Input: part model. Units: mm. Frame: model coordinates. Coordinates: 2 decimals unless noted, no trailing zeros. Loops run counter-clockwise (first coordinate to the right, second up) from the corner with the lowest first, then second, coordinate; pieces in that order, holes last. Notation, with made-up numbers: M -15.5,25 L 16.5,25 A28 ccw 16.5,47 Z; hole C 70,31 d2. An arc over 180 degrees is marked long. Use a Markdown table: item, result. Add a question column.
1. Draft query along Z for faces 1 (the flat face through (-54, 0, 2)), 2 (the cylindrical face through (-75.63, 0.69, 14.27)), 3 (the cylindrical face through (-61.554, 0.69, -13.226)). Return one class per face: +Z half, -Z half, draft (parallel to the pull), parting line (faces both ways), or undercut.
2. Section B-B on x = -63.5. Output: boundary loops of the cut face in (y, z), then the cut area to 3 significant figures.
3. Pin query (flat end, axial travel): pin 1 (1.9 mm diameter, centred on x = -62.65, z = 16.29, fed in from +Y). Return the tip coordinate at first contact, or that it passes through.
4. Line query: L1, parallel to X at y = 1, z = -13; L2, parallel to X at y = 1.2, z = 15; L3, parallel to Z at x = -60, y = 1.35. Output: solid intervals per line, ascending. Write a range as [from, to].
5. Section D-D on z = 21. Output: boundary loops of the cut face in (x, y), then the cut area to 3 significant figures.
6. Section C-C on y = 1.05. Output: boundary loops of the cut face in (x, z), then the cut area to 3 significant figures.
7. Section A-A on z = -14. Output: boundary loops of the cut face in (x, y).
Autodesk Inventor part; units mm, degrees
ref_plane "YZ Plane" through (0, 0, 0) normal (1, 0, 0) x (0, 1, 0)
ref_plane "XZ Plane" through (0, 0, 0) normal (0, 1, 0) x (-1, 0, 0)
ref_plane "XY Plane" through (0, 0, 0) normal (0, 0, 1) x (1, 0, 0)
sketch "Sketch1" plane through (0, 0, 0) normal (0, 1, 0) x (-1, 0, 0)
  line L0 (55.4027, 26.2487) -> (74.9027, 14.9904)
  line L1 (75.9027, 13.2583) -> (75.9027, -9.2583)
  line L2 (74.9027, -10.9904) -> (55.4027, -22.2487)
  line L3 (53.4027, -22.2487) -> (33.9027, -10.9904)
  line L4 (32.9027, -9.2583) -> (32.9027, 13.2583)
  line L5 (33.9027, 14.9904) -> (53.4027, 26.2487)
  arc A0 (33.9027, 14.9904) -> (32.9027, 13.2583) centre (34.9027, 13.2583) ccw
  arc A1 (32.9027, -9.2583) -> (33.9027, -10.9904) centre (34.9027, -9.2583) ccw
  arc A2 (53.4027, -22.2487) -> (55.4027, -22.2487) centre (54.4027, -20.5167) ccw
  arc A3 (74.9027, -10.9904) -> (75.9027, -9.2583) centre (73.9027, -9.2583) ccw
  arc A4 (75.9027, 13.2583) -> (74.9027, 14.9904) centre (73.9027, 13.2583) ccw
  arc A5 (55.4027, 26.2487) -> (53.4027, 26.2487) centre (54.4027, 24.5167) ccw
  circle A6 centre (63.1527, -13.1554) radius 1.6
  circle A7 centre (62.6527, 16.2894) radius 1.6
  point P0 (0, 0)
  point P1 (54.4027, 26.8261)
  point P2 (75.9027, 14.413)
  point P3 (75.9027, -10.413)
  point P4 (54.4027, -22.8261)
  point P5 (32.9027, -10.413)
  point P6 (32.9027, 14.413)
  dimension "d0" = 3.2
  dimension "d1" = 3.2
extrude "Extrusion1" add sketch "Sketch1" along normal blind 1.4
properties part number "Kicker PCB"
Answers below:
| question | item | result |
|---|---|---|
| 1 | face 1 | draft |
| 1 | face 2 | +Z half |
| 1 | face 3 | undercut |
| 2 | outline | M 0,-17.57 L 1.4,-17.57 L 1.4,-14.72 L 0,-14.72 Z; M 0,-11.59 L 1.4,-11.59 L 1.4,14.93 L 0,14.93 Z; M 0,17.65 L 1.4,17.65 L 1.4,21.57 L 0,21.57 Z |
| 2 | area | 46.6 mm² |
| 3 | pin 1 | passes through |
| 4 | L1 | x = [-71.42, -64.75], [-61.56, -37.38] |
| 4 | L2 | x = [-74.89, -63.6], [-61.71, -33.92] |
| 4 | L3 | z = [-19.59, 23.59] |
| 5 | outline | M -64.49,0 L -44.31,0 L -44.31,1.4 L -64.49,1.4 Z |
| 5 | area | 28.3 mm² |
| 6 | outline | M -75.9,-9.26 A2 ccw -74.9,-10.99 L -55.4,-22.25 A2 ccw -53.4,-22.25 L -33.9,-10.99 A2 ccw -32.9,-9.26 L -32.9,13.26 A2 ccw -33.9,14.99 L -53.4,26.25 A2 ccw -55.4,26.25 L -74.9,14.99 A2 ccw -75.9,13.26 Z; hole C -63.15,-13.16 d3.2; hole C -62.65,16.29 d3.2 |
| 6 | area | 1,580 mm² |
| 7 | outline | M -69.69,0 L -64.51,0 L -64.51,1.4 L -69.69,1.4 Z; M -61.79,0 L -39.12,0 L -39.12,1.4 L -61.79,1.4 Z |
